from build123d import *

# Parameters (mm, degrees)
BOSS_EXTRUDE6_DEPTH = 2.7
BOSS_EXTRUDE7_START = 2.7
SKETCH2_4_R         = 4
SKETCH2_4_R_2       = 2.15
BOSS_EXTRUDE7_DEPTH = 1
FILLET1_R           = 1
CUT_EXTRUDE1_START  = 10
SKETCH3_W           = 10
SKETCH3_H           = 2.4
CUT_EXTRUDE1_DEPTH  = 2


with BuildPart() as part:
    # Sketch2 → Boss-Extrude6 (new body)
    with BuildSketch(Plane(origin=(0, 0, 0), x_dir=(1, 0, 0), z_dir=(0, 1, 0))):
        with BuildLine():
            Line((14.35, 4), (0, 4))
            Line((0, 4), (0, -10))
            Line((0, -10), (4.07179677, -10))
            Line((4.07179677, -10), (7.535898385, -4))
            ThreePointArc((7.535898385, -4), (11, -2), (14.464101615, -4))
            Line((14.464101615, -4), (17.92820323, -10))
            Line((17.92820323, -10), (25.35, -10))
            ThreePointArc((25.35, -10), (32.421067812, -7.071067812), (35.35, 0))
            Line((35.35, 0), (35.35, 4))
            Line((35.35, 4), (32.35, 4))
            Line((32.35, 4), (32.35, 0))
            ThreePointArc((32.35, 0), (23.35, -9), (14.35, 0))
            Line((14.35, 0), (14.35, 4))
        make_face()
    extrude(amount=BOSS_EXTRUDE6_DEPTH)

    # Sketch2<4> → Boss-Extrude7 (add)
    # profile 1 of 7: a face of its own
    with BuildSketch(Plane(origin=(0, 0, 0), x_dir=(1, 0, 0), z_dir=(0, 1, 0)).offset(BOSS_EXTRUDE7_START)):
        with BuildLine():
            Line((14.35, 4), (0, 4))
            Line((0, 4), (0, -10))
            Line((0, -10), (4.07179677, -10))
            Line((4.07179677, -10), (7.535898385, -4))
            ThreePointArc((7.535898385, -4), (11, -2), (14.464101615, -4))
            Line((14.464101615, -4), (17.92820323, -10))
            Line((17.92820323, -10), (25.35, -10))
            ThreePointArc((25.35, -10), (32.421067812, -7.071067812), (35.35, 0))
            Line((35.35, 0), (35.35, 4))
            Line((35.35, 4), (32.35, 4))
            Line((32.35, 4), (32.35, 0))
            ThreePointArc((32.35, 0), (23.35, -9), (14.35, 0))
            Line((14.35, 0), (14.35, 4))
        make_face()
    # profile 2 of 7: a face of its own
    with BuildSketch(Plane(origin=(0, 0, 0), x_dir=(1, 0, 0), z_dir=(0, 1, 0)).offset(BOSS_EXTRUDE7_START)):
        with BuildLine():
            Line((7.535898385, -4), (4.07179677, -10))
            Line((4.07179677, -10), (11, -10))
            ThreePointArc((11, -10), (7.535898385, -8), (7.535898385, -4))
        make_face()
    # profile 3 of 7: a face of its own
    with BuildSketch(Plane(origin=(0, 0, 0), x_dir=(1, 0, 0), z_dir=(0, 1, 0)).offset(BOSS_EXTRUDE7_START)):
        with Locations((11, -6)):
            Circle(SKETCH2_4_R)
        with Locations(Location((11, -6, 0), (0, 0, 270))):
            Circle(SKETCH2_4_R_2, mode=Mode.SUBTRACT)
    # profile 4 of 7: a face of its own
    with BuildSketch(Plane(origin=(0, 0, 0), x_dir=(1, 0, 0), z_dir=(0, 1, 0)).offset(BOSS_EXTRUDE7_START)):
        with BuildLine():
            ThreePointArc((15, -6), (13.828427125, -8.828427125), (11, -10))
            Line((11, -10), (17.92820323, -10))
            Line((17.92820323, -10), (14.464101615, -4))
            ThreePointArc((14.464101615, -4), (14.863703305, -4.96472382), (15, -6))
        make_face()
    # profile 5 of 7: a face of its own
    with BuildSketch(Plane(origin=(0, 0, 0), x_dir=(1, 0, 0), z_dir=(0, 1, 0)).offset(BOSS_EXTRUDE7_START)):
        with BuildLine():
            Line((31.412257748, 4), (15.287742252, 4))
            ThreePointArc((15.287742252, 4), (14.587571121, 2.054224947), (14.35, 0))
            ThreePointArc((14.35, 0), (23.35, -9), (32.35, 0))
            ThreePointArc((32.35, 0), (32.112428879, 2.054224947), (31.412257748, 4))
        make_face()
        with Locations(Location((23.35, 0, 0), (0, 0, 270))):
            Circle(SKETCH2_4_R_2, mode=Mode.SUBTRACT)
    # profile 6 of 7: a face of its own
    with BuildSketch(Plane(origin=(0, 0, 0), x_dir=(1, 0, 0), z_dir=(0, 1, 0)).offset(BOSS_EXTRUDE7_START)):
        with BuildLine():
            Line((15.287742252, 4), (14.35, 4))
            Line((14.35, 4), (14.35, 0))
            ThreePointArc((14.35, 0), (14.587571121, 2.054224947), (15.287742252, 4))
        make_face()
    # profile 7 of 7: a face of its own
    with BuildSketch(Plane(origin=(0, 0, 0), x_dir=(1, 0, 0), z_dir=(0, 1, 0)).offset(BOSS_EXTRUDE7_START)):
        with BuildLine():
            Line((32.35, 4), (31.412257748, 4))
            ThreePointArc((31.412257748, 4), (32.112428879, 2.054224947), (32.35, 0))
            Line((32.35, 0), (32.35, 4))
        make_face()
    extrude(amount=BOSS_EXTRUDE7_DEPTH)

    # Mirror1: part across plane


with BuildPart() as part_1:
    add(part.part)
    add(part.part.mirror(Plane.ZX))

    # Mirror2: part across plane


with BuildPart() as part_2:
    add(part_1.part)
    add(part_1.part.mirror(Plane(origin=(0, 0, 0), x_dir=(0, 0, 1), z_dir=(1, 0, 0))))

    # Fillet1
    fillet1_edges = [part_2.edges().sort_by_distance(p)[0] for p in [
        (-35.35, 0, -4),
        (-14.35, 0, -4),
        (-32.35, 0, -4),
        (-17.92820323, 0, 10),
        (-4.07179677, 0, 10),
        (17.92820323, 0, 10),
        (4.07179677, 0, 10),
        (14.35, 0, -4),
        (32.35, 0, -4),
        (35.35, 0, -4),
    ]]
    fillet(fillet1_edges, radius=FILLET1_R)

    # Sketch3 → Cut-Extrude1 (cut)
    with BuildSketch(Plane.XY.offset(CUT_EXTRUDE1_START)):
        Rectangle(SKETCH3_W, SKETCH3_H)
    extrude(amount=-CUT_EXTRUDE1_DEPTH, mode=Mode.SUBTRACT)


solid = part_2.part
Geometry: final body of the model. Coordinates: model frame, mm. A direction names the side the tool comes from. Round coordinates to 2 decimals unless told otherwise and drop trailing zeros. Order: outer loops, then holes, each group sorted by start corner. A loop starts at its lowest first (then second) coordinate and runs counter-clockwise, first axis right, second up.
Q1. Mould query, pull axis Z, two halves, no side actions, for faces 1 (the face through (0, 0, 8)), 2 (the face through (25.48, 3.19, -0.28)), 3 (the face through (0, -3.7, 3)). Classes: released by +Z, released by -Z, zero draft, split by the parting line, or undercut.
Result sheet:
face 1: released by +Z
face 2: undercut
face 3: zero draft
Q2. Pin query (flat end, axial travel): pin 1 (3 mm diameter, centred on x = -26, y = 1, fed in from -Z); pin 2 (1.5 mm diameter, centred on x = 10, y = 0, fed in from +Z); pin 3 (2.5 mm diameter, centred on x = -11, z = 6, fed in from -Y); pin 4 (3 mm diameter, centred on y = -3, z = 8.5, fed in from +X). Return the tip coordinate at first contact, or that it passes through.
Result sheet:
pin 1: stops at z = 7.99
pin 2: stops at z = 2.4
pin 3: passes through
pin 4: stops at x = 32.49
Q3. Access query for faces 4 (the face through (11.09, -3.19, 3.85)), 5 (the face through (-13, -2.7, 8)), 6 (the face through (-32.35, 0, -2)). Directions: +Z, -Z, +X, -X, +Y, -Y. A direction counts if a zero-diameter tool reaches every point of the face in a straight line with its end or side. Return the directions, or none.
Result sheet:
face 4: +Y, -Y
face 5: +Z
face 6: -Z
Q4. Material intervals for probe 1 along X at (y, z) = (3.5, 0); probe 2 along X at (y, z) = (-3, 6); probe 3 along Y at (x, z) = (-19.5, 4), sorted ascending.
Result sheet:
probe 1: x = -35.35 to -25.5, -21.2 to 21.2, 25.5 to 35.35
probe 2: x = -33.35 to -13.15, -8.85 to 8.85, 13.15 to 33.35
probe 3: y = -3.7 to -2.7, 2.7 to 3.7
Q5. Section B-B, the plane z = -1.25. Output: boundary loops of the cut face in (x, y), and give its area (3 significant figures).
Result sheet:
outline: (-35.35, -3.7) - (-25.1, -3.7) - (-25.1, -2.7) - (-32.35, -2.7) - (-32.35, 2.7) - (-25.1, 2.7) - (-25.1, 3.7) - (-35.35, 3.7) - close; (-21.6, -3.7) - (21.6, -3.7) - (21.6, -2.7) - (14.35, -2.7) - (14.35, 2.7) - (21.6, 2.7) - (21.6, 3.7) - (-21.6, 3.7) - (-21.6, 2.7) - (-14.35, 2.7) - (-14.35, -2.7) - (-21.6, -2.7) - close; (25.1, -3.7) - (35.35, -3.7) - (35.35, 3.7) - (25.1, 3.7) - (25.1, 2.7) - (32.35, 2.7) - (32.35, -2.7) - (25.1, -2.7) - close
area: 315 mm2
Q6. Section A-A, the plane x = -11. Output: boundary loops of the cut face in (y, z).
Result sheet:
outline: (-3.7, -4) - (3.7, -4) - (3.7, 3.85) - (2.7, 3.85) - (2.7, 2) - (-2.7, 2) - (-2.7, 3.85) - (-3.7, 3.85) - close; (-3.7, 8.15) - (-2.7, 8.15) - (-2.7, 10) - (-3.7, 10) - close; (2.7, 8.15) - (3.7, 8.15) - (3.7, 10) - (2.7, 10) - close
Q7. Section D-D, the plane z = 6. Give the number of separate pieces and of enclosed holes in the cut face, and give its area (3 significant figures).
Result sheet:
separate pieces: 3
enclosed holes: 2
area: 232 mm2
